```python
from build123d import *

# Parameters (mm, degrees)
SKETCH1_W                                = 203.2
SKETCH1_H                                = 254
SKETCH1_R                                = 33.02
BOSS_EXTRUDE1_DEPTH                      = 5.588
SKETCH7_R                                = 7
CUT_EXTRUDE6_DEPTH                       = 10
CIRPATTERN2_COUNT                        = 3
SKETCH9_R                                = 1.7
CUT_EXTRUDE8_DEPTH                       = 163.735324205
SKETCH10_R                               = 2.665
CUT_EXTRUDE9_DEPTH                       = 498.241984141
CUT_EXTRUDE10_DEPTH                      = 163.735324205
MIRROR1_AT_THE_SECOND_PLANE_COPY_1_DEPTH = 163.735324205


with BuildPart() as part:
    # Sketch1 → Boss-Extrude1 (new body)
    with BuildSketch(Plane.XY):
        Rectangle(SKETCH1_W, SKETCH1_H)
        Circle(SKETCH1_R, mode=Mode.SUBTRACT)
    extrude(amount=BOSS_EXTRUDE1_DEPTH)

    # Sketch7 → Cut-Extrude6 (cut)
    with BuildSketch(Plane(origin=(-207.785981093, -42.996428153, 5.588), x_dir=(0.9999282090774324, -0.011982349151927488, 0), z_dir=(0, 0, 1))):
        with Locations(Location((249.755489637, 45.661901138, 0), (0, 0, 0.686554465))):
            Circle(SKETCH7_R)
    cut_extrude6 = extrude(amount=-CUT_EXTRUDE6_DEPTH, mode=Mode.SUBTRACT)

    # CirPattern2: Cut-Extrude6 ×3 about axis
    cirpattern2_axis = Axis((0, 0, 0), (0, 0, 1))
    for i in range(1, CIRPATTERN2_COUNT):
        add(cut_extrude6.rotate(cirpattern2_axis, i * 360 / CIRPATTERN2_COUNT), mode=Mode.SUBTRACT)

    # Sketch9 → Cut-Extrude8 (cut, through all)
    with BuildSketch(Plane(origin=(0, 0, 0), x_dir=(-1, 0, 0), z_dir=(0, 0, -1))):
        with Locations((37.035546616, -21.139735697)):
            Circle(SKETCH9_R)
        with Locations((37.035546616, -52.139735697)):
            Circle(SKETCH9_R)
        with Locations((6.035546616, -52.139735697)):
            Circle(SKETCH9_R)
    extrude(amount=-CUT_EXTRUDE8_DEPTH, mode=Mode.SUBTRACT)

    # Sketch10 → Cut-Extrude9 (cut, through all)
    with BuildSketch(Plane(origin=(-338.26084164, -104.82063118, 5.588), x_dir=(0.9999190535665993, -0.012723455288419916, 0), z_dir=(0, 0, 1))):
        with Locations(Location((429.565270691, 25.963287337, 0), (0, 0, 0.729019959))):
            Circle(SKETCH10_R)
    extrude(amount=-CUT_EXTRUDE9_DEPTH, mode=Mode.SUBTRACT)

    # Sketch11 → Cut-Extrude10 (cut, through all)
    with BuildSketch(Plane(origin=(0, 0, 0), x_dir=(-1, 0, 0), z_dir=(0, 0, -1))):
        with BuildLine():
            Line((-94.265, -118.11), (-94.265, -105.41))
            ThreePointArc((-94.265, -105.41), (-91.6, -102.745), (-88.935, -105.41))
            Line((-88.935, -105.41), (-88.935, -118.11))
            ThreePointArc((-88.935, -118.11), (-91.6, -120.775), (-94.265, -118.11))
        make_face()
    cut_extrude10 = extrude(amount=-CUT_EXTRUDE10_DEPTH, mode=Mode.SUBTRACT)

    # Mirror1: Cut-Extrude10 across plane
    add(cut_extrude10.mirror(Plane(origin=(0, 0, 0), x_dir=(0, 0, 1), z_dir=(1, 0, 0))), mode=Mode.SUBTRACT)

    # Mirror1 at the second plane: Cut-Extrude10 across plane
    add(cut_extrude10.mirror(Plane.ZX), mode=Mode.SUBTRACT)

    # Mirror1 at the second plane copy 1 sketc → Mirror1 at the second plane copy 1 (cut, through all)
    with BuildSketch(Plane(origin=(0, 0, 0), x_dir=(1, 0, 0), z_dir=(0, 0, -1))):
        with BuildLine():
            Line((-94.265, -118.11), (-94.265, -105.41))
            ThreePointArc((-94.265, -105.41), (-91.6, -102.745), (-88.935, -105.41))
            Line((-88.935, -105.41), (-88.935, -118.11))
            ThreePointArc((-88.935, -118.11), (-91.6, -120.775), (-94.265, -118.11))
        make_face()
    extrude(amount=-MIRROR1_AT_THE_SECOND_PLANE_COPY_1_DEPTH, mode=Mode.SUBTRACT)


solid = part.part
```
For this review, take the finished solid that the model builds, in its own axes (mm). A direction names the side the tool comes from. Coordinates: 2 decimals unless noted, no trailing zeros. Loops run counter-clockwise (first coordinate to the right, second up) from the corner with the lowest first, then second, coordinate; pieces in that order, holes last.
1. Add section B-B, the plane y = 9.5. Give the boundary of the cut face in (x, z).
2. Add section C-C, the plane x = 0. Give the boundary of the cut face in (y, z), then the cut area to 3 significant figures.
3. Add section D-D, the plane z = 1.85. Count the separate pieces of the cut face and the enclosed holes in it, then the cut area to 3 significant figures.
4. Mouldability with a two-part tool opening along Y and no side actions: class faces 1 (the flat face through (21, 30, 0)), 2 (the flat face through (-1, -127, 3)), 3 (the cylindrical face through (-91.541, 120.774, 2.755)) as +Y half, -Y half, draft (parallel to the pull), parting line (faces both ways), or undercut.
5. For line 1 (X direction, y = -108.5, z = 1) (3 decimals); line 2 (Y direction, x = 91.6, z = 1.3) (3 decimals); line 3 (X direction, y = -12, z = 3.85), list the stretches that pass through material, from the lowest coordinate up.
6. Insertion check: P1, Ø7, axis at x = 91.6, y = -84.325, coming from the +Z side; P2, Ø11, axis at x = -20.96, y = 36.97, coming from the +Z side. Each pin has a flat end and moves straight along its axis. Give the tip position at first contact, or say it passes through.
7. Add section A-A, the plane x = -91.6. Give the boundary of the cut face in (y, z) (3 decimals), then the cut area to 3 significant figures.
8. For faces 4 (the flat face through (101.6, -2, 3)), 5 (the cylindrical face through (-91.541, -120.774, 2.755)), list the 3-axis set-ups (+Z, -Z, +X, -X, +Y, -Y) from which the entire face can be reached by the end or side of a thin tool; tool diameter is ignored.
Result:
1. outline: (-101.6, 0) - (-31.62, 0) - (-31.62, 5.59) - (-101.6, 5.59) - close; (31.62, 0) - (101.6, 0) - (101.6, 5.59) - (31.62, 5.59) - close
2. outline: (-127, 0) - (-33.02, 0) - (-33.02, 5.59) - (-127, 5.59) - close; (33.02, 0) - (127, 0) - (127, 5.59) - (33.02, 5.59) - close
2. area: 1,050 mm2
3. separate pieces: 1
3. enclosed holes: 12
3. area: 47,300 mm2
4. face 1: draft
4. face 2: -Y half
4. face 3: undercut
5. line 1: x = -101.6 to -94.265, -88.935 to 88.935, 94.265 to 101.6
5. line 2: y = -127 to -120.775, -102.745 to -86.99, -81.66 to 102.745, 120.775 to 127
5. line 3: x = -101.6 to -30.76, 30.76 to 101.6
6. P1: stops at z = 5.59
6. P2: passes through
7. outline: (-127, 0) - (-120.775, 0) - (-120.775, 5.588) - (-127, 5.588) - close; (-102.745, 0) - (102.745, 0) - (102.745, 5.588) - (-102.745, 5.588) - close; (120.775, 0) - (127, 0) - (127, 5.588) - (120.775, 5.588) - close
7. area: 1,220 mm2
8. face 4: +Z, -Z, +X, +Y, -Y
8. face 5: +Z, -Z
